Autodesk Inventor part; units mm, degrees
ref_plane "YZ Plane" through (0, 0, 0) normal (1, 0, 0) x (0, 1, 0)
ref_plane "XZ Plane" through (0, 0, 0) normal (0, 1, 0) x (-1, 0, 0)
ref_plane "XY Plane" through (0, 0, 0) normal (0, 0, 1) x (1, 0, 0)
sketch "Sketch1" plane through (0, 0, 0) normal (0, 0, 1) x (1, 0, 0)
  line L0 (33.655, 33.655) -> (-33.655, 33.655)
  line L1 (-33.655, 33.655) -> (-33.655, -33.655)
  line L2 (-33.655, -33.655) -> (33.655, -33.655)
  line L3 (33.655, -33.655) -> (33.655, 33.655)
  line L4 (33.655, 33.655) -> (-33.655, -33.655) construction
  line L5 (-33.655, 33.655) -> (33.655, -33.655) construction
  circle A0 centre (0, 0) radius 39.0641 construction
  point P0 (-27.6225, 27.6225)
  point P1 (27.6225, 27.6225)
  point P2 (27.6225, -27.6225)
  point P3 (-27.6225, -27.6225)
  dimension "d1" = 67.31
  dimension "d2" = 67.31
  dimension "d3" = 55.245
extrude "Extrusion1" add sketch "Sketch1" along normal blind 5.08
hole "Hole1" at (-27.6225, 27.6225, 0) at (27.6225, 27.6225, 0) at (27.6225, -27.6225, 0) at (-27.6225, -27.6225, 0) direction (0, 0, 1) diameter 5.08 end through all
sketch "Sketch2" plane through (0, 0, 0) normal (0, 0, -1) x (-1, 0, 0)
  line L0 (33.655, -33.655) -> (-33.655, -33.655)
  line L1 (-16.51, -33.655) -> (-16.51, -43.815)
  line L2 (-16.51, -43.815) -> (1.905, -43.815)
  line L3 (1.905, -43.815) -> (1.905, -33.655)
  line L4 (-33.655, -33.655) -> (-33.655, 33.655)
  line L5 (1.905, -33.655) -> (1.905, -39.243)
  line L6 (1.905, -39.243) -> (33.655, -39.243)
  line L7 (33.655, -39.243) -> (33.655, -33.655)
  line L8 (33.655, 33.655) -> (33.655, -33.655)
  line L9 (33.655, -43.815) -> (-33.655, -43.815) construction
  point P0 (0, 0)
  dimension "d14" = 17.145
  dimension "d16" = 10.16
  dimension "d17" = 4.572
  dimension "d18" = 31.75
extrude "Extrusion2" add sketch "Sketch2" against normal blind 55.88
sketch "Sketch3" plane through (-1.905, -33.655, 0) normal (0, -1, 0) x (1, 0, 0)
  line L0 (0, 0) -> (0, 55.88)
  line L1 (0, 55.88) -> (18.415, 55.88)
  point P0 (1.905, 0)
  point P1 (6.35, 43.18)
  dimension "d21" = 6.35
  dimension "d22" = 12.7
hole "Hole2" at (4.445, -33.655, 43.18) direction (0, -1, 0) diameter 4.572 end through all counterbore diameter 8.89 counterbore depth 5.08
properties part number "Battery Switch Mount"
The model under review builds one solid part; all positions refer to its coordinate system, in mm. A direction names the side the tool comes from. Round coordinates to 2 decimals unless told otherwise and drop trailing zeros. Write each loop counter-clockwise with the first axis right and the second up, starting at its lowest first coordinate (ties: lowest second). Pieces come first, ordered by that corner, then holes. Notation, with made-up numbers: (-23.5, 72.5) - (-13.5, 72.5) arc R10 cw to (-13.5, 91.5) - close; hole circle Ø1 at (75, 2). An arc over 180 degrees is marked (long way). Use one line per item in the form item = value.
Q1. Consider section C-C (x = 14.5). State the section outline as (y, z) points (3 decimals), and give its area (3 significant figures).
Answer key:
outline = (-43.815, 0) - (33.655, 0) - (33.655, 5.08) - (-33.655, 5.08) - (-33.655, 55.88) - (-43.815, 55.88) - close
area = 910 mm2
Q2. Consider section B-B (y = -27). State the section outline as (x, z) points (3 decimals), and give its area (3 significant figures).
Answer key:
outline = (-33.655, 0) - (-30.085, 0) - (-30.085, 5.08) - (-33.655, 5.08) - close; (-25.16, 0) - (25.16, 0) - (25.16, 5.08) - (-25.16, 5.08) - close; (30.085, 0) - (33.655, 0) - (33.655, 5.08) - (30.085, 5.08) - close
area = 292 mm2
Q3. Consider section D-D (z = 32). State the section outline as (x, y) points (3 decimals).
Answer key:
outline = (-33.655, -39.243) - (-1.905, -39.243) - (-1.905, -43.815) - (16.51, -43.815) - (16.51, -33.655) - (-33.655, -33.655) - close
Q4. Draft analysis for pull direction Y (two halves, no side actions). For faces 4 (the flat face through (-3, -38, 55.88)), 5 (the cylindrical face through (-26.65, -25.276, 2.576)), 6 (the flat face through (2, -38.735, 42)), state which applies: +Y half, -Y half, draft (parallel to the pull), parting line (faces both ways), or undercut.
Answer key:
face_4 = draft
face_5 = undercut
face_6 = +Y half
Q5. Consider section A-A (z = 43.18). State the section outline as (x, y) points (3 decimals).
Answer key:
outline = (-33.655, -39.243) - (-1.905, -39.243) - (-1.905, -43.815) - (2.159, -43.815) - (2.159, -38.735) - (0, -38.735) - (0, -33.655) - (-33.655, -33.655) - close; (6.731, -43.815) - (16.51, -43.815) - (16.51, -33.655) - (8.89, -33.655) - (8.89, -38.735) - (6.731, -38.735) - close
Q6. Insertion check: pin 1 Ø12 at (x, y) = (12, -11) entering from +Z; pin 2 Ø7.5 at (x, z) = (4.445, 43.18) entering from +Y (3 decimals); pin 3 Ø4 at (x, y) = (27.62, 27.62) entering from +Z; pin 4 Ø1.5 at (x, z) = (-14, 21) entering from -Y. Each pin has a flat end and moves straight along its axis. Give the tip position at first contact, or say it passes through.
Answer key:
pin_1 = 5.08
pin_2 = -38.735
pin_3 = through
pin_4 = -39.24
Q7. Tool access review of faces 1 (the flat face through (-18, -39.243, 28)), 2 (the flat face through (25, -33.655, 3)), 3 (the flat face through (-9, -33.655, 30)): name each direction out of +Z, -Z, +X, -X, +Y, -Y from which nothing blocks a thin tool from reaching the whole face with its end or side.
Answer key:
face_1 = +Z, -Z, -X, -Y
face_2 = +Z, -Z, +X, -Y
face_3 = +Z, +X, -X, +Y
Q8. For line 1 (Z direction, x = -2, y = 28.5); line 2 (Y direction, x = -5.5, z = 29.5) (3 decimals); line 3 (X direction, y = -40, z = 43) (3 decimals), list the stretches that pass through material, from the lowest coordinate up. Write a range as [from, to].
Answer key:
line_1 = [0, 5.08]
line_2 = [-39.243, -33.655]
line_3 = [-1.905, 2.166], [6.724, 16.51]
